Part model, mm, in its own coordinate system. A direction names the side the tool comes from. Give positions to 0.01 mm unless a question says otherwise; leave off trailing zeros. Order: outer loops, then holes, each group sorted by start corner. A loop starts at its lowest first (then second) coordinate and runs counter-clockwise, first axis right, second up. Notation, with made-up numbers: (-19.75, 82) - (33.25, 82) arc R26 ccw to (33.25, 112) - close; hole circle Ø11 at (45, 24). An arc over 180 degrees is marked (long way). Use a Markdown table: item, result. Add a question column.
Solid Edge part; units mm, degrees
sketch "Sketch1" plane through (0, 0, 0) normal (1, 0, 0) x (0, 1, 0)
  line L0 (42, 40) -> (42, -40)
  line L1 (42, -40) -> (-42, -40)
  line L2 (-42, -40) -> (-42, 40)
  line L3 (-42, 40) -> (42, 40)
extrude "Protrusion1" add sketch "Sketch1" along normal blind 2
sketch "Sketch2" plane through (0, 0, 0) normal (1, 0, 0) x (0, 1, 0)
  line L0 (-42, 38) -> (-25, 38)
  line L1 (-25, 38) -> (-25, 40)
  line L2 (-25, 40) -> (-42, 40)
  line L3 (-42, 40) -> (-42, 38)
  line L4 (-5, 40) -> (-15, 40)
  line L5 (-15, 40) -> (-15, 38)
  line L6 (-15, 38) -> (-5, 38)
  line L7 (-5, 38) -> (-5, 40)
  line L8 (15, 40) -> (5, 40)
  line L9 (5, 40) -> (5, 38)
  line L10 (5, 38) -> (15, 38)
  line L11 (15, 38) -> (15, 40)
  line L12 (42, 40) -> (25, 40)
  line L13 (25, 40) -> (25, 38)
  line L14 (25, 38) -> (42, 38)
  line L15 (42, 38) -> (42, 40)
  line L16 (38, 25) -> (38, 15)
  line L17 (38, 15) -> (40, 15)
  line L18 (40, 15) -> (40, 25)
  line L19 (40, 25) -> (38, 25)
  line L20 (38, 5) -> (38, -5)
  line L21 (38, -5) -> (40, -5)
  line L22 (40, -5) -> (40, 5)
  line L23 (40, 5) -> (38, 5)
  line L24 (38, -15) -> (38, -25)
  line L25 (38, -25) -> (40, -25)
  line L26 (40, -25) -> (40, -15)
  line L27 (40, -15) -> (38, -15)
  line L28 (42, -38) -> (25, -38)
  line L29 (25, -38) -> (25, -40)
  line L30 (25, -40) -> (42, -40)
  line L31 (42, -40) -> (42, -38)
  line L32 (15, -38) -> (5, -38)
  line L33 (5, -38) -> (5, -40)
  line L34 (5, -40) -> (15, -40)
  line L35 (15, -40) -> (15, -38)
  line L36 (-5, -38) -> (-15, -38)
  line L37 (-15, -38) -> (-15, -40)
  line L38 (-15, -40) -> (-5, -40)
  line L39 (-5, -40) -> (-5, -38)
  line L40 (-25, -38) -> (-42, -38)
  line L41 (-42, -38) -> (-42, -40)
  line L42 (-42, -40) -> (-25, -40)
  line L43 (-25, -40) -> (-25, -38)
  line L44 (-38, -25) -> (-38, -15)
  line L45 (-38, -15) -> (-40, -15)
  line L46 (-40, -15) -> (-40, -25)
  line L47 (-40, -25) -> (-38, -25)
  line L48 (-38, 5) -> (-40, 5)
  line L49 (-40, 5) -> (-40, -5)
  line L50 (-40, -5) -> (-38, -5)
  line L51 (-38, -5) -> (-38, 5)
  line L52 (-40, 15) -> (-38, 15)
  line L53 (-38, 15) -> (-38, 25)
  line L54 (-38, 25) -> (-40, 25)
  line L55 (-40, 25) -> (-40, 15)
extrude "Cutout1" cut sketch "Sketch2" along normal blind 2
properties material "Acrylic, high impact grade"
1. Cut at A-A (z = 17). Write the cut outline in (x, y), plus the area to 3 significant figures.
2. Mould opens along Z. For faces 1 (the face through (1, 39, 25)), 2 (the face through (1, 25, 39)), 3 (the face through (1, 33, 38)) say: released by +Z, released by -Z, zero draft, split by the parting line, or undercut.
3. Pin check, flat tips, straight feed: P1, Ø0.6, axis at x = 1, y = -38.5, coming from the +Z side; P2, Ø0.6, axis at x = 1, z = 38.5, coming from the -Y side; P3, Ø0.6, axis at x = 1, z = -39, coming from the +Y side; P4, Ø12, axis at y = 32.5, z = -22.5, coming from the -X side. Stop position of each tip, or through.
4. Tool access for faces 4 (the face through (1, 15, 39)), 5 (the face through (1, -39, 5)), 6 (the face through (1, 5, -39)): list every direction of +Z, -Z, +X, -X, +Y, -Y with a clear straight run to the whole face (end or side of a thin tool).
5. Drill centre lines: probe 1 along Y at (x, z) = (1.2, 4); probe 2 along Z at (x, y) = (1.25, 28). Where is each one in solid material? Low to high. Write a range as [from, to].
6. Cut at B-B (x = 0.55). State how many separate pieces and enclosed holes the cut face has, plus the area to 3 significant figures.
7. Cut at C-C (y = -28.5). Write the cut outline in (x, z), plus the area to 3 significant figures.
Responses:
| question | item | result |
|---|---|---|
| 1 | outline | (0, -42) - (2, -42) - (2, -40) - (0, -40) - close; (0, -38) - (2, -38) - (2, 38) - (0, 38) - close; (0, 40) - (2, 40) - (2, 42) - (0, 42) - close |
| 1 | area | 160 mm² |
| 2 | face 1 | undercut |
| 2 | face 2 | zero draft |
| 2 | face 3 | released by +Z |
| 3 | P1 | stops at z = 38 |
| 3 | P2 | stops at y = -25 |
| 3 | P3 | stops at y = 25 |
| 3 | P4 | stops at x = 0 |
| 4 | face 4 | +Z, +X, -X |
| 4 | face 5 | +X, -X |
| 4 | face 6 | -Z, +X, -X |
| 5 | probe 1 | y = [-42, -40], [-38, 38], [40, 42] |
| 5 | probe 2 | z = [-38, 38] |
| 6 | separate pieces | 1 |
| 6 | enclosed holes | 6 |
| 6 | area | 6,380 mm² |
| 7 | outline | (0, -38) - (2, -38) - (2, 38) - (0, 38) - close |
| 7 | area | 152 mm² |
